Part print with two shaded views. Sizes in mm from the minimum x, y, z corner. Give positions to 0.01 mm unless a question says otherwise; leave off trailing zeros. Order: outer loops, then holes, each group sorted by start corner. A loop starts at its lowest first (then second) coordinate and runs counter-clockwise, first axis right, second up. Notation, with made-up numbers: M -2.5,-9 L 29.5,-9 A13 cw 29.5,4 Z; hole C 46.25,44 d9. An arc over 180 degrees is marked long. Return JSON: item names as keys, results as strings. Group by question number.
1. Pin check, flat tip, straight feed: pin 1 (2 mm diameter, centred on x = 22.5, z = 50, fed in from -Y). Stop position of the tip, or through.
2. Slice it at A-A on z = 68. List the corners of the cut face in (x, y) (1 decimal).
3. Wall check: probe 1 along Z at (x, y) = (44, 0.9) (1 decimal); probe 2 along X at (y, z) = (0.55, 80.5) (1 decimal); probe 3 along Z at (x, y) = (107, 0.3) (1 decimal). Give the ranges that are in metal, low to high. Write a range as [from, to].
4. Slice it at D-D on z = 130. List the corners of the cut face in (x, y) (1 decimal).
5. Slice it at C-C on x = 20.5. List the corners of the cut face in (y, z).
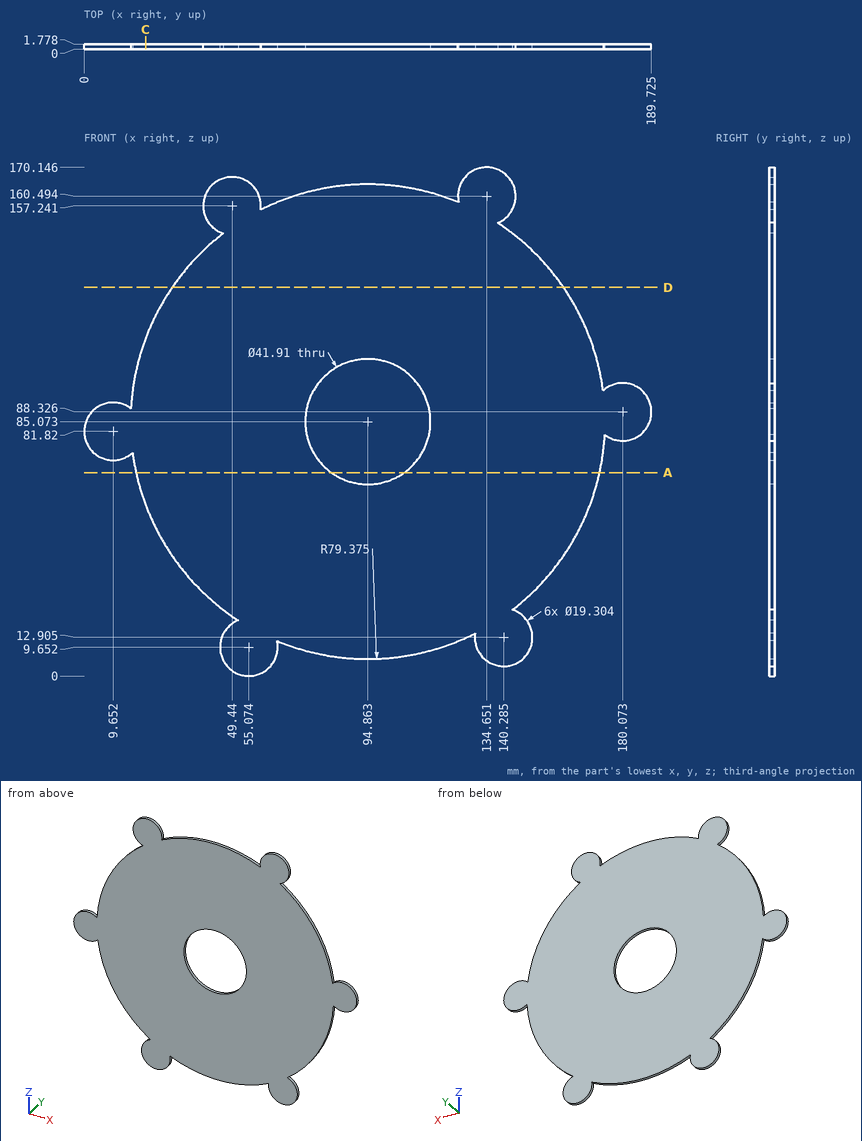
Result:
{
 "1": {"pin 1": "passes through"},
 "2": {"outline": "M 17.3,0 L 82.7,0 L 82.7,1.8 L 17.3,1.8 Z; M 107,0 L 172.4,0 L 172.4,1.8 L 107,1.8 Z"},
 "3": {"probe 1": "z = [24.1, 146], [149.3, 165.2]", "probe 2": "x = [0.1, 74.4], [115.3, 174.1], [174.4, 185.7]", "probe 3": "z = [6.6, 68], [102.2, 163.5]"},
 "4": {"outline": "M 29.4,0 L 160.3,0 L 160.3,1.8 L 29.4,1.8 Z"},
 "5": {"outline": "M 0,57.31 L 1.78,57.31 L 1.78,112.83 L 0,112.83 Z"}
}
